```python
from build123d import *

# Parameters (mm, degrees)
F1_DEPTH  = 11.6
F3_R      = 3
F4_DEPTH  = 3.2
F6_R      = 6
F7_DEPTH  = 5.8
F9_R      = 18.5
F10_DEPTH = 24
F12_R     = 16
F13_DEPTH = 19.3
F14_R     = 1.75
F15_DEPTH = 4


# Not quite as in the source:
# - after a boolean that leaves OpenCascade's solid faulty, fix() repairs it


with BuildPart() as f1:
    # F0 (on Front) → F1 (new body)
    with BuildSketch(Plane.XZ):
        with BuildLine():
            Line((1.8648056199, 2.35), (-1.8648056199, 2.35))
            ThreePointArc((-1.8648056199, 2.35), (0, -3), (1.8648056199, 2.35))
        make_face()
    extrude(amount=-F1_DEPTH)

    # F3 (on offset) → F4 (join)
    with BuildSketch(Plane(origin=(0, 11.6, 0), x_dir=(-1, 0, 0), z_dir=(0, 1, 0))):
        Circle(F3_R)
    extrude(amount=F4_DEPTH)

    # F6 (on offset) → F7 (join)
    with BuildSketch(Plane(origin=(0, 14.8, 0), x_dir=(-1, 0, 0), z_dir=(0, 1, 0))):
        Circle(F6_R)
    extrude(amount=F7_DEPTH)

    add(f1.part.fix(), mode=Mode.REPLACE)

    # F9 (on offset) → F10 (join)
    with BuildSketch(Plane(origin=(0, 20.6, 0), x_dir=(-1, 0, 0), z_dir=(0, 1, 0))):
        with Locations((0, -6.7)):
            Circle(F9_R)
    extrude(amount=F10_DEPTH)

    # F12 (on offset) → F13 (join)
    with BuildSketch(Plane(origin=(0, 44.6, 0), x_dir=(-1, 0, 0), z_dir=(0, 1, 0))):
        with Locations((0, -6.7)):
            Circle(F12_R)
    extrude(amount=F13_DEPTH)

    # F14 (on offset) → F15 (cut)
    with BuildSketch(Plane(origin=(0, 20.6, 0), x_dir=(-1, 0, 0), z_dir=(0, 1, 0))):
        with Locations((-15.15, -6.7)):
            Circle(F14_R)
        with Locations((15.15, -6.7)):
            Circle(F14_R)
        with Locations((7.4, -19.9197768514)):
            Circle(F14_R)
        with Locations((-7.4, -19.9197768514)):
            Circle(F14_R)
        with Locations((-7.4, 6.5197768514)):
            Circle(F14_R)
        with Locations((7.4, 6.5197768514)):
            Circle(F14_R)
    extrude(amount=F15_DEPTH, mode=Mode.SUBTRACT)


solid = f1.part
```
Can you work these out from the model? Positions are in its coordinate system, mm. A direction names the side the tool comes from. Round coordinates to 2 decimals unless told otherwise and drop trailing zeros. Order: outer loops, then holes, each group sorted by start corner. A loop starts at its lowest first (then second) coordinate and runs counter-clockwise, first axis right, second up.
(1) If we section it at D-D (z = 0): Please give me the cut outline in (x, y), plus the area to 3 significant figures.
Results are:
outline: (-17.24, 20.6) - (-6, 20.6) - (-6, 14.8) - (-3, 14.8) - (-3, 0) - (3, 0) - (3, 14.8) - (6, 14.8) - (6, 20.6) - (17.24, 20.6) - (17.24, 44.6) - (14.53, 44.6) - (14.53, 63.9) - (-14.53, 63.9) - (-14.53, 44.6) - (-17.24, 44.6) - close
area: 1,550 mm2
(2) On a 3-axis mill with a long thin cutter (end or side, diameter ignored), from which of +Z, -Z, +X, -X, +Y, -Y can I reach the whole of each face in a straight line? I mean faces 1 (the face through (0, 6, 2.35)), 2 (the face through (0, 63.9, -6)), 3 (the face through (4.01, 32.43, -24.76)), 4 (the face through (5.6, 44.6, 8.5)), 5 (the face through (-8.341, 22.572, 7.995)). Say none if no direction works.
Results are:
face 1: +Z, +X, -X, -Y
face 2: +Z, -Z, +X, -X, +Y
face 3: +Y, -Y
face 4: +Y
face 5: -Y
(3) If I drill on L1, parallel to Z at x = -7, y = 23; L2, parallel to Y at x = 6.5, z = -18; L3, parallel to X at y = 22, z = -6, over which ranges is the centre line in solid material (lowest first)?
Results are:
L1: z = -23.82 to -21.62, -18.22 to 4.82, 8.22 to 10.42
L2: y = 20.6 to 63.9
L3: x = -18.49 to -16.75, -13.55 to 13.55, 16.75 to 18.49
(4) If we section it at C-C (y = 8): Please give me the cut outline in (x, z), plus the area to 3 significant figures.
Results are:
outline: (-1.86, 2.35) arc R3 ccw (long way) to (1.86, 2.35) - close
area: 26.6 mm2
(5) If we section it at A-A (z = -6.7): Please give me the cut outline in (x, y), plus the area to 3 significant figures.
Results are:
outline: (-18.5, 20.6) - (-16.9, 20.6) - (-16.9, 24.6) - (-13.4, 24.6) - (-13.4, 20.6) - (13.4, 20.6) - (13.4, 24.6) - (16.9, 24.6) - (16.9, 20.6) - (18.5, 20.6) - (18.5, 44.6) - (16, 44.6) - (16, 63.9) - (-16, 63.9) - (-16, 44.6) - (-18.5, 44.6) - close
area: 1,480 mm2
(6) I'm going to push flat-ended pins straight in: pin 1 (10 mm diameter, centred on y = 26, z = -14.5, fed in from +X); pin 2 (1.9 mm diameter, centred on x = -1, y = 6, fed in from +Z); pin 3 (5.5 mm diameter, centred on x = -7.4, z = 6.52, fed in from -Y). Where does each tip first touch, or does it pass through?
Results are:
pin 1: stops at x = 18.29
pin 2: stops at z = 2.35
pin 3: stops at y = 20.6
(7) If we section it at B-B (x = 0): Please give me the cut outline in (y, z).
Results are:
outline: (0, -3) - (14.8, -3) - (14.8, -6) - (20.6, -6) - (20.6, -25.2) - (44.6, -25.2) - (44.6, -22.7) - (63.9, -22.7) - (63.9, 9.3) - (44.6, 9.3) - (44.6, 11.8) - (20.6, 11.8) - (20.6, 6) - (14.8, 6) - (14.8, 3) - (11.6, 3) - (11.6, 2.35) - (0, 2.35) - close
(8) We'd pull the mould along X, two halves only. Please class faces 6 (the face through (7.628, 22.572, -18.185)), 7 (the face through (8.69, 22.57, 7.7)), 8 (the face through (0, 0, 0)), 9 (the face through (6, 18, 0)): +X half, -X half, draft (parallel to the pull), parting line (faces both ways), or undercut.
Results are:
face 6: undercut
face 7: undercut
face 8: draft
face 9: parting line
